from build123d import *

# Parameters (mm, degrees)
EXTRUDE_2_DEPTH     = 16
SKETCH_2_R          = 15.5
CUT_EXTRUDE_3_DEPTH = 965.699401752


with BuildPart() as part:
    # 草图1 → 拉伸2 (new body)
    with BuildSketch(Plane.XY):
        Polygon((693.325362834, 420), (83.325362834, 420), (-91.674637166, 0), (-91.674637166, -260), (868.325362834, -260), (868.325362834, 0), align=None)
    extrude(amount=EXTRUDE_2_DEPTH)

    # 草图2 → 拉伸3 (cut, through all)
    with BuildSketch(Plane.XY.offset(16)):
        with Locations((328.325362834, 340)):
            Circle(SKETCH_2_R)
        with Locations((228.325362834, 340)):
            Circle(SKETCH_2_R)
        with Locations((128.325362834, 340)):
            Circle(SKETCH_2_R)
        with Locations(Location((128.325362834, 150, 0), (0, 0, 180))):
            Circle(SKETCH_2_R)
        with Locations(Location((228.325362834, 150, 0), (0, 0, 180))):
            Circle(SKETCH_2_R)
        with Locations(Location((328.325362834, 150, 0), (0, 0, 180))):
            Circle(SKETCH_2_R)
        with Locations((293.325362834, -185)):
            Circle(SKETCH_2_R)
        with Locations((293.325362834, 15)):
            Circle(SKETCH_2_R)
        with Locations((293.325362834, -85)):
            Circle(SKETCH_2_R)
        with Locations((639.758349024, -27.804790016)):
            Circle(SKETCH_2_R)
        with Locations((721.084382293, -116.043536113)):
            Circle(SKETCH_2_R)
        with Locations((802.410415562, -204.28228221)):
            Circle(SKETCH_2_R)
        with Locations((735.570581969, -21.095392271)):
            Circle(SKETCH_2_R)
        with Locations((706.598182617, -210.991679954)):
            Circle(SKETCH_2_R)
        with Locations(Location((625.272149348, -122.752933857, 0), (0, 0, 180))):
            Circle(SKETCH_2_R)
        with Locations(Location((816.896615238, -109.334138368, 0), (0, 0, 180))):
            Circle(SKETCH_2_R)
        with Locations((151.37857632, -122.752933857)):
            Circle(SKETCH_2_R)
        with Locations(Location((70.052543051, -210.991679954, 0), (0, 0, 180))):
            Circle(SKETCH_2_R)
        with Locations(Location((-25.759689894, -204.28228221, 0), (0, 0, 180))):
            Circle(SKETCH_2_R)
        with Locations(Location((55.566343375, -116.043536113, 0), (0, 0, 180))):
            Circle(SKETCH_2_R)
        with Locations(Location((136.892376644, -27.804790016, 0), (0, 0, 180))):
            Circle(SKETCH_2_R)
        with Locations((-40.24588957, -109.334138368)):
            Circle(SKETCH_2_R)
        with Locations(Location((41.080143699, -21.095392271, 0), (0, 0, 180))):
            Circle(SKETCH_2_R)
        with Locations((448.325362834, 150)):
            Circle(SKETCH_2_R)
        with Locations((548.325362834, 150)):
            Circle(SKETCH_2_R)
        with Locations((648.325362834, 150)):
            Circle(SKETCH_2_R)
        with Locations(Location((648.325362834, 340, 0), (0, 0, 180))):
            Circle(SKETCH_2_R)
        with Locations(Location((548.325362834, 340, 0), (0, 0, 180))):
            Circle(SKETCH_2_R)
        with Locations(Location((448.325362834, 340, 0), (0, 0, 180))):
            Circle(SKETCH_2_R)
        with Locations(Location((483.325362834, -85, 0), (0, 0, 180))):
            Circle(SKETCH_2_R)
        with Locations(Location((483.325362834, 15, 0), (0, 0, 180))):
            Circle(SKETCH_2_R)
        with Locations(Location((483.325362834, -185, 0), (0, 0, 180))):
            Circle(SKETCH_2_R)
    extrude(amount=-CUT_EXTRUDE_3_DEPTH, mode=Mode.SUBTRACT)


solid = part.part
Build history of the part. All positions in model axes, mm. Coordinates: 2 decimals unless noted, no trailing zeros. Order: outer loops, then holes, each group sorted by start corner. A loop starts at its lowest first (then second) coordinate and runs counter-clockwise, first axis right, second up. Notation, with made-up numbers: M 75.5,-3.75 L 115.5,-3.75 A10 ccw 115.5,2.25 Z; hole C 19,76.5 d5. An arc over 180 degrees is marked long. One line per question, with ' | ' between items. Start each with the question number.
Q1. Flat gauge pins, fed straight in: pin 1 Ø5 at (y, z) = (287.5, 12.5) entering from -X; pin 2 Ø2 at (y, z) = (156.5, 8) entering from -X; pin 3 Ø25 at (x, y) = (-40.25, -109.33) entering from +Z; pin 4 Ø5 at (y, z) = (248, 6.5) entering from -X. Where does each tip first touch, or does it go through?
Q2. Saw through at D-D (z = 4). Count the separate pieces of the cut face and the enclosed holes in it, then the cut area to 3 significant figures.
Q3. Saw through at A-A (y = 15). List the corners of the cut face in (x, z), then the cut area to 3 significant figures.
Q4. Saw through at B-B (y = 340). List the corners of the cut face in (x, z).
Q5. Saw through at C-C (y = 150). List the corners of the cut face in (x, z).
Q6. Probe L1, parallel to Y at x = 484, z = 1.75; L2, parallel to Y at x = 661.5, z = 9.5; L3, parallel to Y at x = 125, z = 3. List the from-to ranges inside material, lowest first. Write a range as from..to.
Q7. Two-plate mould, pull along Y, no slides. Class faces 1 (the face through (113.541, 145.344, 8.112)), 2 (the face through (382, 85, 0)), 3 (the face through (-2.95, 212.94, 7.89)), 4 (the face through (281, -194.4, 8.1)): +Y half, -Y half, draft (parallel to the pull), parting line (faces both ways), or undercut.
Check values:
1) pin 1: stops at x = 27.08 | pin 2: stops at x = -26.88 | pin 3: passes through | pin 4: stops at x = 10.62
2) separate pieces: 1 | enclosed holes: 32 | area: 555,000 mm2
3) outline: M -85.42,0 L 277.83,0 L 277.83,16 L -85.42,16 Z; M 308.83,0 L 467.83,0 L 467.83,16 L 308.83,16 Z; M 498.83,0 L 862.08,0 L 862.08,16 L 498.83,16 Z | area: 14,200 mm2
4) outline: M 49.99,0 L 112.83,0 L 112.83,16 L 49.99,16 Z; M 143.83,0 L 212.83,0 L 212.83,16 L 143.83,16 Z; M 243.83,0 L 312.83,0 L 312.83,16 L 243.83,16 Z; M 343.83,0 L 432.83,0 L 432.83,16 L 343.83,16 Z; M 463.83,0 L 532.83,0 L 532.83,16 L 463.83,16 Z; M 563.83,0 L 632.83,0 L 632.83,16 L 563.83,16 Z; M 663.83,0 L 726.66,0 L 726.66,16 L 663.83,16 Z
5) outline: M -29.17,0 L 112.83,0 L 112.83,16 L -29.17,16 Z; M 143.83,0 L 212.83,0 L 212.83,16 L 143.83,16 Z; M 243.83,0 L 312.83,0 L 312.83,16 L 243.83,16 Z; M 343.83,0 L 432.83,0 L 432.83,16 L 343.83,16 Z; M 463.83,0 L 532.83,0 L 532.83,16 L 463.83,16 Z; M 563.83,0 L 632.83,0 L 632.83,16 L 563.83,16 Z; M 663.83,0 L 805.83,0 L 805.83,16 L 663.83,16 Z
6) L1: y = -260..-200.49, -169.51..-100.49, -69.51..-0.49, 30.49..420 | L2: y = -260..141.83, 158.17..331.83, 348.17..420 | L3: y = -260..-37.75, -17.86..134.86, 165.14..324.86, 355.14..420
7) face 1: undercut | face 2: draft | face 3: +Y half | face 4: undercut
